Autodesk Inventor part; units mm, degrees
ref_plane "YZ Plane" through (0, 0, 0) normal (1, 0, 0) x (0, 1, 0)
ref_plane "XZ Plane" through (0, 0, 0) normal (0, 1, 0) x (-1, 0, 0)
ref_plane "XY Plane" through (0, 0, 0) normal (0, 0, 1) x (1, 0, 0)
sketch "Sketch1" plane through (0, 0, 0) normal (0, 1, 0) x (-1, 0, 0)
  line L0 (-35, 36.5) -> (35, 36.5)
  line L1 (35, 36.5) -> (35, -36.5)
  line L2 (35, -36.5) -> (-35, -36.5)
  line L3 (-35, -36.5) -> (-35, 36.5)
  line L4 (-35, 36.5) -> (35, -36.5) construction
  line L5 (35, 36.5) -> (-35, -36.5) construction
  line L6 (-35, -36.5) -> (-35, -50.5)
  line L7 (-35, -50.5) -> (-6, -50.5)
  line L8 (6.0499, -50.5) -> (35, -50.5)
  line L9 (35, -50.5) -> (35, -36.5)
  line L10 (6.0499, -36.5) -> (6.0499, -43.5)
  line L11 (6.0499, -43.5) -> (-6, -43.5)
  line L12 (-6, -43.5) -> (-6, -36.5)
  line L13 (-6, -50.5) -> (-6, -43.5)
  line L14 (6.0499, -50.5) -> (6.0499, -43.5)
  point P0 (0, 0)
  dimension "d0" = 70
  dimension "d1" = 73
  dimension "d2" = 14
  dimension "d3" = 29
  dimension "d4" = 7
  dimension "d5" = 87
  dimension "d61" = 7
  dimension "d64" = 12.0499
sketch "Sketch2" plane through (0, 0, 0) normal (0, 1, 0) x (-1, 0, 0)
  point P0 (0, 0)
extrude "Extrusion1" add sketch "Sketch1" along normal blind 8 contours L0 L1 L2 L3 | L2 L12 L13 L7 L6 | L9 L8 L14 L10 L2
sketch "Sketch3" plane through (0, 8, 0) normal (0, 1, 0) x (1, 0, 0)
  line L0 (9, 36) -> (9, -36.5)
  line L1 (35, -36.5) -> (35, 36)
  line L2 (9, 36) -> (35, 36)
  line L3 (6, 50.5) -> (6, 36.5)
  line L4 (-9.0499, -36.5) -> (-9.0499, 35.5)
  line L5 (-9.0499, 35.5) -> (-35, 35.5)
  line L6 (-35, 35.5) -> (-35, -36.5)
  line L7 (-35, -36.5) -> (-9.0499, -36.5)
  line L8 (-6.0499, 36.5) -> (-6.0499, 50.5)
  line L9 (9, -36.5) -> (35, -36.5)
  point P0 (0, 0)
  point P1 (6, 43.5)
  point P2 (-6.0499, 43.5)
  dimension "d8" = 3
  dimension "d9" = 3
extrude "Extrusion2" cut sketch "Sketch3" against normal blind 2.61
sketch "Sketch4" plane through (0, 0, 0) normal (0, -1, 0) x (1, 0, 0)
  line L0 (-35, 36.5) -> (35, 36.5)
  line L1 (-29.525, 36.5) -> (-29.525, -42.6114)
  line L2 (-35, -50.5) -> (-35, 36.5)
  line L3 (29.525, 36.5) -> (29.525, -43.7753)
  line L4 (35, 36.5) -> (35, -50.5)
  line L5 (-14.525, 36.5) -> (-14.525, -22.6051)
  line L6 (14.5, 36.5) -> (14.5, -47.1695)
  line L7 (-22.025, 36.5) -> (-22.025, -33.1573)
  line L8 (-22.025, 36.5) -> (-22.025, 23.3)
  circle A0 centre (-22.025, 21.55) radius 1.75
  line L9 (-9.0499, 36.5) -> (9, 36.5)
  line L10 (22, 36.5) -> (22, -38.3698)
  line L11 (22, 36.5) -> (22, 23.3)
  circle A1 centre (22, 21.55) radius 1.75
  circle A2 centre (22, -18.45) radius 1.75
  circle A3 centre (-22.025, -18.45) radius 1.75
  point P0 (0, 0)
  point P1 (-35, -56.5)
  point P2 (22.1782, -20.1909)
  point P3 (-23.772, -18.5519)
  dimension "d40" = 3.5
  dimension "d45" = 3.5
  dimension "d46" = 3.5
  dimension "d47" = 36.5
  dimension "d48" = 3.5
  dimension "d31" = 5.475
  dimension "d32" = 5.475
  dimension "d33" = 15
  dimension "d38" = 7.5
  dimension "d39" = 13.2
  dimension "d43" = 7.5
  dimension "d44" = 13.2
  dimension "d49" = 40
  dimension "d57" = 14.525
hole "Hole1" at (22, 0, 21.55) at (22, 0, -18.45) at (-22.025, 0, 21.55) at (-22.025, 0, -18.45) direction (0, 1, 0) diameter 3.5 depth 15.664 counterbore diameter 10 counterbore depth 2
sketch "Sketch5" plane through (6, 0, -36.5) normal (0, 0, -1) x (-1, 0, 0)
  line L0 (41, 0) -> (-29, 0)
  line L1 (0, 0) -> (15.0499, 0)
  line L2 (15.0499, 0) -> (15.0499, 8)
  line L3 (15.0499, 8) -> (0, 8)
  line L4 (0, 8) -> (0, 0)
  point P0 (6, 0)
extrude "Extrusion3" add sketch "Sketch5" along normal blind 0.5
sketch "Sketch10" plane through (0, 0, 0) normal (0, -1, 0) x (1, 0, 0)
  line L0 (-7.6499, -30) -> (-7.6499, 26.5)
  line L1 (-7.6499, 26.5) -> (7.6, 26.5)
  line L2 (7.6, 26.5) -> (7.6, -30)
  line L3 (7.6, -30) -> (-7.6499, -30)
  line L4 (6, -37) -> (-6.0499, -37)
  line L5 (-35, 36.5) -> (35, 36.5)
  line L6 (9, 36.5) -> (9, -36)
  line L7 (-9.0499, -35.5) -> (-9.0499, 36.5)
  point P0 (0, 0)
  dimension "d72" = 7
  dimension "d73" = 10
  dimension "d74" = 1.4
  dimension "d75" = 1.4
extrude "Extrusion4" cut sketch "Sketch10" against normal blind 7
sketch "Sketch12" plane through (6, 0, -37) normal (0, 0, -1) x (-1, 0, 0)
  line L0 (12.0499, 0) -> (12.0499, 8)
  line L1 (0, 0) -> (0, 8)
  circle A0 centre (3.025, 4) radius 1.5
  circle A1 centre (9.025, 4) radius 1.5
  line L2 (6.025, 1.0105) -> (6.025, 8)
  line L3 (12.0499, 8) -> (0, 8)
  point P0 (6, 0)
  dimension "d78" = 12.0499
  dimension "d79" = 3
  dimension "d80" = 3
  dimension "d82" = 3
  dimension "d83" = 3
  dimension "d84" = 2.5
hole "Hole2" at (2.975, 4, -37) at (-3.025, 4, -37) direction (0, 0, 1) diameter 3 depth 10.5 tip angle 118
sketch "Sketch13" plane through (0, 8, 0) normal (0, 1, 0) x (1, 0, 0)
  line L0 (-7.6499, -26.5) -> (7.6, -26.5)
  line L1 (-7.7014, -26.5) -> (7.6, -26.5)
  line L2 (7.6, -26.5) -> (7.6, 7.4212)
  line L3 (7.6, -26.5) -> (7.6, 30)
  line L4 (-7.6499, 7.4212) -> (-7.6499, -26.5)
  line L5 (-7.6499, 7.4212) -> (7.6, 7.4212)
  point P0 (0, 0)
  point P1 (8.2986, -26.5)
extrude "Extrusion5" cut sketch "Sketch13" against normal blind 10
properties part number "floor-4" material "ABS Plastic"
Design review of the part built by this model. Coordinates are the model's own, in mm. A direction names the side the tool comes from. Give positions to 0.01 mm unless a question says otherwise; leave off trailing zeros. Loops run counter-clockwise (first coordinate to the right, second up) from the corner with the lowest first, then second, coordinate; pieces in that order, holes last. Notation, with made-up numbers: (43.5, 4.25) -> (73.5, 4.25) arc R21 cw to (73.5, 17.25) -> close; hole circle Ø6 at (28.5, -15). An arc over 180 degrees is marked (long way). One line per question, with ' | ' between items. Start each with the question number.
(1) We need section A-A (z = -5). State the section outline as (x, y) points, and give its area (3 significant figures).
(2) We need section C-C (y = 3.75). State the section outline as (x, z) points (3 decimals).
(3) We need section D-D (z = -18.45). State the section outline as (x, y) points (3 decimals).
(4) Insertion check: P1, Ø1.3, axis at y = 7, z = 5.5, coming from the +X side; P2, Ø3, axis at x = -20, z = -18, coming from the -Y side; P3, Ø3, axis at x = 4.5, z = 8, coming from the -Y side; P4, Ø13, axis at x = 22, z = 2.5, coming from the +Y side. Each pin has a flat end and moves straight along its axis. Give the tip position at first contact, or say it passes through.
(5) For line 1 (X direction, y = 4, z = -33) (3 decimals); line 2 (X direction, y = 3.2, z = -18.45) (3 decimals); line 3 (Z direction, x = 22, y = 3.75), list the stretches that pass through material, from the lowest coordinate up.
(6) Draft analysis for pull direction X (two halves, no side actions). For faces 5 (the face through (-2.45, 5.386, -33.451)), 6 (the face through (0, 3, 36.5)), 7 (the face through (-35, 3, -6)), state which applies: +X half, -X half, draft (parallel to the pull), parting line (faces both ways), or undercut.
(7) For faces 1 (the face through (-22, 5.39, 0)), 2 (the face through (-6.05, 4, -44)), 3 (the face through (25.04, 1.01, -14.48)), 4 (the face through (0, 4, 26.5)), list the 3-axis set-ups (+Z, -Z, +X, -X, +Y, -Y) from which the entire face can be reached by the end or side of a thin tool; tool diameter is ignored.
(8) We need section B-B (x = 22). State the section outline as (y, z) points.
The answers:
1) outline: (-35, 0) -> (-7.65, 0) -> (-7.65, 8) -> (-9.05, 8) -> (-9.05, 5.39) -> (-35, 5.39) -> close; (7.6, 0) -> (35, 0) -> (35, 5.39) -> (9, 5.39) -> (9, 8) -> (7.6, 8) -> close | area: 302 mm^2
2) outline: (-35, -50.5) -> (-6.05, -50.5) -> (-6.05, -37) -> (-4.504, -37) -> (-4.504, -30) -> (-7.65, -30) -> (-7.65, 26.5) -> (7.6, 26.5) -> (7.6, -30) -> (4.454, -30) -> (4.454, -37) -> (6, -37) -> (6, -50.5) -> (35, -50.5) -> (35, 36.5) -> (-35, 36.5) -> close; (-1.546, -37) -> (1.496, -37) -> (1.496, -30) -> (-1.546, -30) -> close; hole circle Ø3.5 at (-22.025, -18.45); hole circle Ø3.5 at (-22.025, 21.55); hole circle Ø3.5 at (22, -18.45); hole circle Ø3.5 at (22, 21.55)
3) outline: (-35, 0) -> (-27.025, 0) -> (-27.025, 2) -> (-23.775, 2) -> (-23.775, 5.39) -> (-35, 5.39) -> close; (-20.275, 2) -> (-17.025, 2) -> (-17.025, 0) -> (-7.65, 0) -> (-7.65, 7) -> (7.6, 7) -> (7.6, 0) -> (17, 0) -> (17, 2) -> (20.25, 2) -> (20.25, 5.39) -> (9, 5.39) -> (9, 8) -> (-9.05, 8) -> (-9.05, 5.39) -> (-20.275, 5.39) -> close; (23.75, 2) -> (27, 2) -> (27, 0) -> (35, 0) -> (35, 5.39) -> (23.75, 5.39) -> close
4) P1: stops at x = 9 | P2: stops at y = 2 | P3: passes through | P4: stops at y = 5.39
5) line 1: x = -35 to -4.525, -1.525 to 1.475, 4.475 to 35 | line 2: x = -35 to -23.775, -20.275 to -7.65, 7.6 to 20.25, 23.75 to 35 | line 3: z = -50.5 to -20.2, -16.7 to 19.8, 23.3 to 36.5
6) face 5: undercut | face 6: draft | face 7: -X half
7) face 1: +Z, -X, +Y | face 2: -Z, +Y, -Y | face 3: -Y | face 4: +Y, -Y
8) outline: (0, -50.5) -> (8, -50.5) -> (8, -36) -> (5.39, -36) -> (5.39, -20.2) -> (2, -20.2) -> (2, -23.45) -> (0, -23.45) -> close; (0, -13.45) -> (2, -13.45) -> (2, -16.7) -> (5.39, -16.7) -> (5.39, 19.8) -> (2, 19.8) -> (2, 16.55) -> (0, 16.55) -> close; (0, 26.55) -> (2, 26.55) -> (2, 23.3) -> (5.39, 23.3) -> (5.39, 36.5) -> (0, 36.5) -> close
